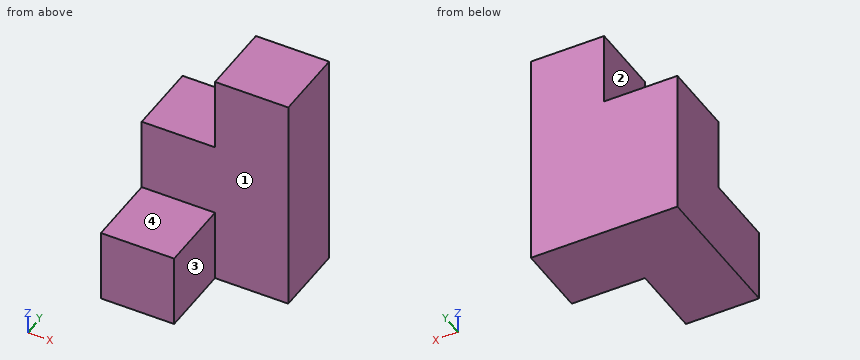
```python
from build123d import *

# Parameters (mm, degrees)
F0_W     = 19.05
F0_H     = 19.05
F1_DEPTH = 19.05
F2_DEPTH = 19.05
F3_DEPTH = 38.1


with BuildPart() as f1:
    # F0 (on Front) → F1 (new body)
    with BuildSketch(Plane.XZ):
        with Locations((-12.501768, 27.558763)):
            Rectangle(F0_W, F0_H)
    extrude(amount=F1_DEPTH)

    # F0 (on Front) → F2 (join)
    with BuildSketch(Plane.XZ):
        Polygon((-22.026768, -1.016237), (-22.026768, -20.066237), (-2.976768, -20.066237), (-2.976768, 18.033763), (-22.026768, 18.033763), (-41.076768, 18.033763), (-41.076768, -1.016237), align=None)
    extrude(amount=F2_DEPTH)

    # F0 (on Front) → F3 (join)
    with BuildSketch(Plane.XZ):
        with Locations((-31.551768, -10.541237)):
            Rectangle(F0_W, F0_H)
    extrude(amount=F3_DEPTH)


solid = f1.part
```
Can you work these out from the model? Positions are in its coordinate system, mm. Face numbers are marked on the shaded views. A direction names the side the tool comes from. Coordinates: 2 decimals unless noted, no trailing zeros. Loops run counter-clockwise (first coordinate to the right, second up) from the corner with the lowest first, then second, coordinate; pieces in that order, holes last.
1) Imagine slicing it at C-C on x = -15.5. List the corners of the cut face in (y, z) for me, plus the area to 3 significant figures.
2) Imagine slicing it at A-A on y = -14. List the corners of the cut face in (x, z) for me.
3) Imagine slicing it at D-D on z = 30.5. List the corners of the cut face in (x, y) for me, plus the area to 3 significant figures.
4) Imagine slicing it at B-B on z = -13. List the corners of the cut face in (x, y) for me, plus the area to 3 significant figures.
5) For pin 1 (15 mm diameter, centred on x = -28, y = -30, fed in from +Z); pin 2 (5 mm diameter, centred on x = -24, z = 20, fed in from -Y); pin 3 (10 mm diameter, centred on x = -31.5, y = -19.5, fed in from +Z), each with a flat end and sliding along its axis, tell me the tip position at first contact or that it passes through.
6) Which directions (+Z, -Z, +X, -X, +Y, -Y) give clear straight access to the entire face, cutting with the end or side of a thin tool? Please do the marked faces 1, 2, 3 and 4.
7) I need wall thicknesses on probe 1 along Y at (x, z) = (-20.5, 14); probe 2 along Z at (x, y) = (-35, -27); probe 3 along X at (y, z) = (-13, 28). Which ranges of each line are inside material? Lowest first, please.
Completed:
1. outline: (-19.05, -20.07) - (0, -20.07) - (0, 37.08) - (-19.05, 37.08) - close
1. area: 1,090 mm2
2. outline: (-41.08, -20.07) - (-2.98, -20.07) - (-2.98, 37.08) - (-22.03, 37.08) - (-22.03, 18.03) - (-41.08, 18.03) - close
3. outline: (-22.03, -19.05) - (-2.98, -19.05) - (-2.98, 0) - (-22.03, 0) - close
3. area: 363 mm2
4. outline: (-41.08, -38.1) - (-22.03, -38.1) - (-22.03, -19.05) - (-2.98, -19.05) - (-2.98, 0) - (-41.08, 0) - close
4. area: 1,090 mm2
5. pin 1: stops at z = -1.02
5. pin 2: stops at y = -19.05
5. pin 3: stops at z = 18.03
6. face 1: +Z, +X, -Y
6. face 2: +Z, -X, +Y, -Y
6. face 3: +Z, -Z, +X, -Y
6. face 4: +Z, +X, -X, -Y
7. probe 1: y = -19.05 to 0
7. probe 2: z = -20.07 to -1.02
7. probe 3: x = -22.03 to -2.98
